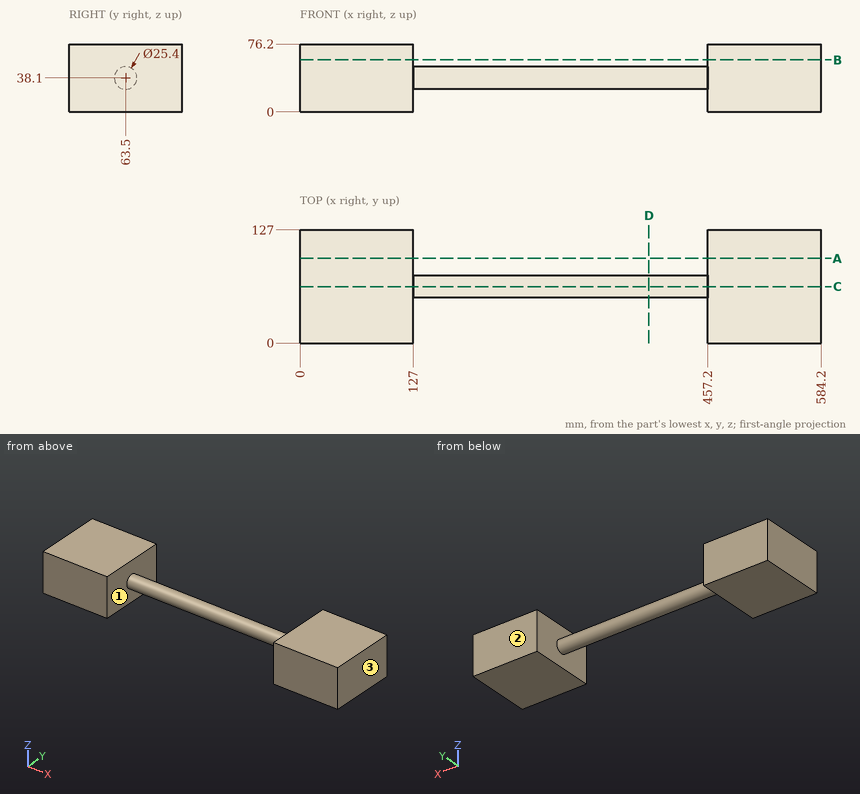
Answer from the drawing. Dimensions are ordinates in mm from the lowest x, y and z of the part. Round coordinates to 2 decimals unless told otherwise and drop trailing zeros. Order: outer loops, then holes, each group sorted by start corner. A loop starts at its lowest first (then second) coordinate and runs counter-clockwise, first axis right, second up.
1) Straight lines are drawn through the part: L1, parallel to X at y = 38.5, z = 58.5; L2, parallel to Y at x = 163, z = 37.5; L3, parallel to Z at x = 369.5, y = 54. For each, find the intervals that lie inside material, in ascending order.
2) Flat-ended cylindrical pins translate along their axes: pin 1 (3 mm diameter, centred on x = 201.5, z = 29.5, fed in from -Y); pin 2 (12 mm diameter, centred on x = 91.5, z = 12.5, fed in from -Y). Find the tip coordinate at first contact, or state that the pin passes through.
3) The part is cut by section B-B on z = 58.5. Write down the section's boundary in (x, y).
4) The part is cut by section C-C on y = 63.5. Write down the section's boundary in (x, z).
5) The part is cut by section A-A on y = 95. Write down the section's boundary in (x, z), plus the area to 3 significant figures.
6) The mould has two halves that part along X. Classify the marked faces 1, 2 and 3: released by +X, released by -X, zero draft, split by the parting line, or undercut.
7) The part is cut by section D-D on x = 391. Write down the section's boundary in (y, z).
Resolved:
1. L1: x = 0 to 127, 457.2 to 584.2
1. L2: y = 50.81 to 76.19
1. L3: z = 29.67 to 46.53
2. pin 1: stops at y = 52.97
2. pin 2: stops at y = 0
3. outline: (0, 0) - (127, 0) - (127, 127) - (0, 127) - close; (457.2, 0) - (584.2, 0) - (584.2, 127) - (457.2, 127) - close
4. outline: (0, 0) - (127, 0) - (127, 25.4) - (457.2, 25.4) - (457.2, 0) - (584.2, 0) - (584.2, 76.2) - (457.2, 76.2) - (457.2, 50.8) - (127, 50.8) - (127, 76.2) - (0, 76.2) - close
5. outline: (0, 0) - (127, 0) - (127, 76.2) - (0, 76.2) - close; (457.2, 0) - (584.2, 0) - (584.2, 76.2) - (457.2, 76.2) - close
5. area: 19,400 mm2
6. face 1: undercut
6. face 2: zero draft
6. face 3: released by +X
7. outline: circle Ø25.4 at (63.5, 38.1)
